Input: part model. Units: mm. Frame: model coordinates. Face numbers are marked on the shaded views. A direction names the side the tool comes from. Give positions to 0.01 mm unless a question says otherwise; leave off trailing zeros. Loops run counter-clockwise (first coordinate to the right, second up) from the corner with the lowest first, then second, coordinate; pieces in that order, holes last. Notation, with made-up numbers: (68.25, 21) -> (106.25, 21) arc R25 ccw to (106.25, 50) -> close; hole circle Ø6 at (-40, 13). An arc over 180 degrees is marked (long way). One line per question, with ' | ' between items.
from build123d import *

# Parameters (mm, degrees)
F0_W      = 1066.8
F0_H      = 558.8
F0_W_2    = 1028.7
F0_H_2    = 520.7
F1_DEPTH  = 38.1
F2_W      = 1028.7
F2_H      = 6.35
F3_DEPTH  = 520.7
F4_W      = 952.5
F4_H      = 19.05
F5_DEPTH  = 63.5
F6_W      = 63.5
F6_H      = 406.4
F7_DEPTH  = 63.5
F8_W      = 19.05
F8_H      = 88.9
F9_DEPTH  = 406.4
F10_W     = 914.4
F10_H     = 19.05
F11_DEPTH = 190.5
F12_W     = 812.8
F12_H     = 1.27
F13_DEPTH = 12.7
F14_W     = 266.7
F14_H     = 1.27
F15_DEPTH = 952.5
F16_W     = 19.05
F16_H     = 62.23
F17_DEPTH = 952.5


with BuildPart() as f1:
    # F0 (on Top) → F1 (new body)
    with BuildSketch(Plane.XY):
        Rectangle(F0_W, F0_H)
        Rectangle(F0_W_2, F0_H_2, mode=Mode.SUBTRACT)
    extrude(amount=F1_DEPTH)

    # F2 (on face) → F3 (join)
    with BuildSketch(Plane(origin=(0, -260.35, 0), x_dir=(-1, 0, 0), z_dir=(0, 1, 0))):
        with Locations((0, 31.75)):
            Rectangle(F2_W, F2_H)
    extrude(amount=F3_DEPTH)

    # F4 (on face) → F5 (join)
    with BuildSketch(Plane(origin=(0, 0, 28.575), x_dir=(1, 0, 0), z_dir=(0, 0, -1))):
        with Locations((0, 212.725)):
            Rectangle(F4_W, F4_H)
    extrude(amount=F5_DEPTH)

    # F6 (on face) → F7 (join)
    with BuildSketch(Plane(origin=(0, 0, 28.575), x_dir=(1, 0, 0), z_dir=(0, 0, -1))):
        with Locations((-412.75, 0)):
            Rectangle(F6_W, F6_H)
        with Locations((412.75, 0)):
            Rectangle(F6_W, F6_H)
    extrude(amount=F7_DEPTH)

    # F8 (on face) → F9 (join)
    with BuildSketch(Plane(origin=(0, 0, 28.575), x_dir=(1, 0, 0), z_dir=(0, 0, -1))):
        Polygon((-406.4, 241.3), (-495.3, 241.3), (-495.3, 222.25), (-476.25, 222.25), (-406.4, 222.25), align=None)
        with Locations((-485.775, 177.8)):
            Rectangle(F8_W, F8_H)
        with Locations((-485.775, -177.8)):
            Rectangle(F8_W, F8_H)
        Polygon((-476.25, -222.25), (-495.3, -222.25), (-495.3, -241.3), (-406.4, -241.3), (-406.4, -222.25), align=None)
        Polygon((476.25, -222.25), (406.4, -222.25), (406.4, -241.3), (495.3, -241.3), (495.3, -222.25), align=None)
        with Locations((485.775, -177.8)):
            Rectangle(F8_W, F8_H)
        Polygon((495.3, 241.3), (406.4, 241.3), (406.4, 222.25), (476.25, 222.25), (495.3, 222.25), align=None)
        with Locations((485.775, 177.8)):
            Rectangle(F8_W, F8_H)
    extrude(amount=F9_DEPTH)

    # F10 (on face) → F11 (join)
    with BuildSketch(Plane(origin=(0, 0, 28.575), x_dir=(1, 0, 0), z_dir=(0, 0, -1))):
        Polygon((476.25, -222.25), (476.25, 203.2), (457.2, 203.2), (457.2, -203.2), (457.2, -222.25), align=None)
        with Locations((0, -212.725)):
            Rectangle(F10_W, F10_H)
        Polygon((-457.2, -222.25), (-457.2, -203.2), (-457.2, 203.2), (-476.25, 203.2), (-476.25, -222.25), align=None)
    extrude(amount=F11_DEPTH)

    # F12 (on face) → F13 (cut)
    with BuildSketch(Plane(origin=(0, 222.25, 0), x_dir=(-1, 0, 0), z_dir=(0, 1, 0))):
        with Locations((0, -35.56)):
            Rectangle(F12_W, F12_H)
        with Locations((0, -99.06)):
            Rectangle(F12_W, F12_H)
    extrude(amount=-F13_DEPTH, mode=Mode.SUBTRACT)

    # F14 (on face) → F15 (cut)
    with BuildSketch(Plane(origin=(-476.25, 0, 0), x_dir=(0, -1, 0), z_dir=(-1, 0, 0))):
        with Locations((0, -35.56)):
            Rectangle(F14_W, F14_H)
        with Locations((0, -100.33)):
            Rectangle(F14_W, F14_H)
    extrude(amount=-F15_DEPTH, mode=Mode.SUBTRACT)

    # F16 (on face) → F17 (join)
    with BuildSketch(Plane.YZ.offset(-476.25)):
        with Locations((-212.725, -130.81)):
            Rectangle(F16_W, F16_H)
        with Locations((-212.725, -67.31)):
            Rectangle(F16_W, F16_H)
    extrude(amount=F17_DEPTH)


solid = f1.part
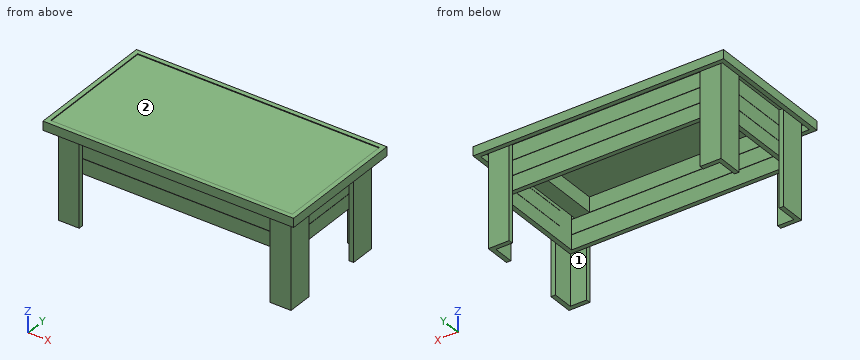
1. Ray query, line 1 along X through (y, z) = (149, 13.5); line 2 along X through (y, z) = (-69, -20); line 3 along Y through (x, z) = (-411, -260). Return the intervals inside material, ascending. Write a range as from..to.
Determined:
line 1: x = -533.4..-514.35, -495.3..-457.2, -444.5..-381, 381..444.5, 457.2..495.3, 514.35..533.4 | line 2: x = -476.25..-457.2, -444.5..-381, 381..444.5, 457.2..476.25 | line 3: y = -241.3..-222.25, 222.25..241.3
2. Pin query (flat end, axial travel): P1, Ø16, axis at y = 222, z = -130, coming from the +X side; P2, Ø8, axis at y = -87.5, z = -121.5, coming from the -X side; P3, Ø21, axis at x = -467.5, y = 1.5, coming from the -Z side (3 decimals). Return the tip coordinate at first contact, or that it passes through.
Determined:
P1: stops at x = 495.3 | P2: stops at x = -476.25 | P3: stops at z = -161.925
3. Section query C-C (z = -15). Count the separate pieces of the cut face and the enclosed holes in it, then the cut area to 3 significant figures.
Determined:
separate pieces: 1 | enclosed holes: 3 | area: 117,000 mm2
4. Section query D-D (z = -116). Output: boundary loops of the cut face in (x, y), then the cut area to 3 significant figures.
Determined:
outline: (-495.3, -241.3) -> (-406.4, -241.3) -> (-406.4, -222.25) -> (406.4, -222.25) -> (406.4, -241.3) -> (495.3, -241.3) -> (495.3, -133.35) -> (476.25, -133.35) -> (476.25, 133.35) -> (495.3, 133.35) -> (495.3, 241.3) -> (406.4, 241.3) -> (406.4, 222.25) -> (-406.4, 222.25) -> (-406.4, 241.3) -> (-495.3, 241.3) -> (-495.3, 133.35) -> (-476.25, 133.35) -> (-476.25, -133.35) -> (-495.3, -133.35) -> close; hole (-457.2, -203.2) -> (457.2, -203.2) -> (457.2, 203.2) -> (-457.2, 203.2) -> close | area: 65,300 mm2
5. Reachability of the marked faces 1 and 2 from +Z, -Z, +X, -X, +Y, -Y: full face, straight path, thin tool, end or side. Return the list, or none.
Determined:
face 1: -Z | face 2: +Z
6. Section query A-A (z = -248.5). Output: boundary loops of the cut face in (x, y), then the cut area to 3 significant figures.
Determined:
outline: (-495.3, -241.3) -> (-406.4, -241.3) -> (-406.4, -222.25) -> (-476.25, -222.25) -> (-476.25, -133.35) -> (-495.3, -133.35) -> close; (-495.3, 133.35) -> (-476.25, 133.35) -> (-476.25, 222.25) -> (-406.4, 222.25) -> (-406.4, 241.3) -> (-495.3, 241.3) -> close; (406.4, -241.3) -> (495.3, -241.3) -> (495.3, -133.35) -> (476.25, -133.35) -> (476.25, -222.25) -> (406.4, -222.25) -> close; (406.4, 222.25) -> (476.25, 222.25) -> (476.25, 133.35) -> (495.3, 133.35) -> (495.3, 241.3) -> (406.4, 241.3) -> close | area: 13,500 mm2
